Autodesk Inventor part; units mm, degrees
ref_plane "YZ Plane" through (0, 0, 0) normal (1, 0, 0) x (0, 1, 0)
ref_plane "XZ Plane" through (0, 0, 0) normal (0, 1, 0) x (-1, 0, 0)
ref_plane "XY Plane" through (0, 0, 0) normal (0, 0, 1) x (1, 0, 0)
sketch "Esboço2" plane through (0, 0, 0) normal (0, 0, 1) x (1, 0, 0)
  line L0 (-1.4393, 191.951) -> (-2.5, 191.951) construction
  line L1 (-2.5, 191.951) -> (-2.5, 190.8903) construction
  line L2 (67.4393, -37.951) -> (68.5, -37.951) construction
  line L3 (68.5, -37.951) -> (68.5, -36.8903) construction
  line L4 (-2.5, 191.951) -> (68.5, 191.951)
  line L5 (68.5, 191.951) -> (68.5, -37.951)
  line L6 (68.5, -37.951) -> (-2.5, -37.951)
  line L7 (-2.5, -37.951) -> (-2.5, 191.951)
  point P0 (0, 0)
  dimension "d14" = 71
extrude "Extrusão2" add sketch "Esboço2" along normal blind 9.5
sketch "Esboço3" plane through (0, 0, 9.5) normal (0, 0, 1) x (1, 0, 0)
  point P0 (0, 0)
  point P1 (41.8302, -5)
  point P2 (24.1698, -5)
  point P3 (41.8302, -33)
  point P4 (24.1698, -33)
  point P5 (54.985, 104.9)
  point P6 (11.015, 104.9)
  point P7 (5, 61.2)
  point P8 (61, 61.2)
hole "Furo1" at (11.015, 104.9, 9.5) at (54.985, 104.9, 9.5) at (5, 61.2, 9.5) at (61, 61.2, 9.5) at (24.1698, -5, 9.5) at (41.8302, -5, 9.5) at (24.1698, -33, 9.5) at (41.8302, -33, 9.5) direction (0, 0, -1) diameter 4 end through all counterbore diameter 9 counterbore depth 5.5
properties part number "suporte_cabeça_superior"
Verification items for the finished model (mm, model axes). A direction names the side the tool comes from. Give positions to 0.01 mm unless a question says otherwise; leave off trailing zeros. Loops run counter-clockwise (first coordinate to the right, second up) from the corner with the lowest first, then second, coordinate; pieces in that order, holes last. Notation, with made-up numbers: (13, 9.5) - (59, 9.5) arc R32 ccw to (59, 41.5) - close; hole circle Ø2 at (0, -18.75). An arc over 180 degrees is marked (long way). Write item = value, one per line. Start each with the question number.
Q1. Depth check by flat-ended pin: P1, Ø6.5, axis at x = 24.17, y = -5, coming from the +Z side. Enter the tip coordinate at first touch or a pass-through.
Q2. Mould release check, pull along Y, two halves, no side actions. Record for faces 3 (the face through (62, 59, 4)), 4 (the face through (33, -37.951, 5)), 5 (the face through (33, 79, 0)): released by +Y, released by -Y, zero draft, split by the parting line, or undercut.
Q3. Tool access check on faces 1 (the face through (44, -34, 4)), 2 (the face through (4.399, 59.292, 1.972)). Record the directions out of +Z, -Z, +X, -X, +Y, -Y that give a thin tool (end or side, any length) a straight path to the whole face; none if there is none.
Q4. Thickness scan on line 1 (X direction, y = -33, z = 2.75); line 2 (X direction, y = -33, z = 8.05); line 3 (Y direction, x = 61, z = 1.05). Record the ranges inside material, lowest first.
Q5. Cross-section at A-A, the plane y = 61.2. Enter the section's corners in (x, z), and give its area (4 significant figures).
Q6. Cross-section at B-B, the plane z = 7.75. State how many separate pieces and enclosed holes the cut face has, and give its area (3 significant figures).
Answer key:
q1.P1 = 4
q2.face_3 = undercut
q2.face_4 = released by -Y
q2.face_5 = zero draft
q3.face_1 = +Z
q3.face_2 = +Z, -Z
q4.line_1 = -2.5 to 22.17, 26.17 to 39.83, 43.83 to 68.5
q4.line_2 = -2.5 to 19.67, 28.67 to 37.33, 46.33 to 68.5
q4.line_3 = -37.95 to 59.2, 63.2 to 191.95
q5.outline = (-2.5, 0) - (3, 0) - (3, 4) - (0.5, 4) - (0.5, 9.5) - (-2.5, 9.5) - close; (7, 0) - (59, 0) - (59, 4) - (56.5, 4) - (56.5, 9.5) - (9.5, 9.5) - (9.5, 4) - (7, 4) - close; (63, 0) - (68.5, 0) - (68.5, 9.5) - (65.5, 9.5) - (65.5, 4) - (63, 4) - close
q5.area = 543.5 mm^2
q6.separate_pieces = 1
q6.enclosed_holes = 8
q6.area = 15,800 mm^2
